Geometry check sheet. Reference: the model listing, model coordinates, mm. A direction names the side the tool comes from. Round coordinates to 2 decimals unless told otherwise and drop trailing zeros. Write each loop counter-clockwise with the first axis right and the second up, starting at its lowest first coordinate (ties: lowest second). Pieces come first, ordered by that corner, then holes.
Item 1: Depth check by flat-ended pin: P1, Ø11.5, axis at x = 80, y = 40, coming from the -Z side; P2, Ø8, axis at x = 72.5, z = 55.5, coming from the -Y side; P3, Ø5, axis at x = 78.5, y = 39.5, coming from the +Z side; P4, Ø13.5, axis at x = 59, y = 77.5, coming from the +Z side. Enter the tip coordinate at first touch or a pass-through.
Item 2: Scan lines: probe 1 along Y at (x, z) = (7, 20.5); probe 2 along Z at (x, y) = (41, 37); probe 3 along Z at (x, y) = (87.5, 22). Record each from-to range of solid material in increasing order.
Item 3: Cross-section at B-B (x = 26). Enter the section's corners in (y, z).
Item 4: Cross-section at A-A (y = 20). Enter the section's corners in (x, z), then the cut area to 4 significant figures.
Item 5: Access from +Z, -Z, +X, -X, +Y, -Y to the whole of each face (thin tool, end or side, straight path). Record for faces 1 (the face through (6.349, 44.957, 15.14)), 2 (the face through (45, 40, 25)), 3 (the face through (60, 20, 13)), 4 (the face through (20, 84, 55)).
Item 6: Draft check along Y on faces 5 (the face through (42.83, 30.24, 15.45)), 6 (the face through (89.619, 18.085, 39.79)), 7 (the face through (80, 0, 13)), 8 (the face through (85, 20, 55)). Enter one of: pulls with the +Y half, pulls with the -Y half, needs draft (parallel to the pull), parting line crosses it, or undercut.
Item 7: Cross-section at D-D (y = 38.5). Enter the section's corners in (x, z), then the cut area to 3 significant figures.
Item 8: Cross-section at C-C (z = 63). Enter the section's corners in (x, y), then the cut area to 3 significant figures.
from build123d import *

# Parameters (mm, degrees)
F1_DEPTH  = 100
F2_R      = 5
F3_DEPTH  = 30
F4_R      = 5
F5_DEPTH  = 20
F6_W      = 60
F6_H      = 40
F7_DEPTH  = 95
F8_W      = 45
F8_H      = 40
F9_DEPTH  = 25
F10_R     = 15
F11_DEPTH = 15
F12_R     = 10
F13_DEPTH = 25


with BuildPart() as f1:
    # F0 (on Right) → F1 (new body)
    with BuildSketch(Plane.YZ):
        Polygon((0, 25), (0, 0), (100, 0), (100, 100), (60, 25), align=None)
    extrude(amount=F1_DEPTH)

    # F2 (on face) → F3 (join)
    with BuildSketch(Plane.XY.offset(25)):
        with Locations((85, 20)):
            Circle(F2_R)
    extrude(amount=F3_DEPTH)

    # F4 (on face) → F5 (cut)
    with BuildSketch(Plane.XY.offset(25)):
        with Locations((7, 40)):
            Circle(F4_R)
        with Locations((80, 40)):
            Circle(F4_R)
    extrude(amount=-F5_DEPTH, mode=Mode.SUBTRACT)

    # F6 (on Front) → F7 (cut)
    with BuildSketch(Plane.XZ):
        with Locations((50, 60)):
            Rectangle(F6_W, F6_H)
    extrude(amount=-F7_DEPTH, mode=Mode.SUBTRACT)

    # F8 (on face) → F9 (cut)
    with BuildSketch(Plane.XY.offset(25)):
        with Locations((37.5, 20)):
            Rectangle(F8_W, F8_H)
    extrude(amount=-F9_DEPTH, mode=Mode.SUBTRACT)

    # F10 (on face) → F11 (cut)
    with BuildSketch(Plane.XY.offset(25)):
        with Locations((45, 40)):
            Circle(F10_R)
    extrude(amount=-F11_DEPTH, mode=Mode.SUBTRACT)

    # F12 (on face) → F13 (join)
    with BuildSketch(Plane.XY.offset(25)):
        with Locations((45, 40)):
            Circle(F12_R)
    extrude(amount=-F13_DEPTH)


solid = f1.part
Resolved:
1. P1: stops at z = 0
1. P2: stops at y = 95
1. P3: stops at z = 5
1. P4: stops at z = 40
2. probe 1: y = 0 to 35, 45 to 100
2. probe 2: z = 0 to 25
2. probe 3: z = 0 to 55
3. outline: (40, 0) - (100, 0) - (100, 100) - (89.33, 80) - (95, 80) - (95, 40) - (68, 40) - (60, 25) - (40, 25) - close
4. outline: (0, 0) - (15, 0) - (15, 25) - (0, 25) - close; (60, 0) - (100, 0) - (100, 25) - (90, 25) - (90, 55) - (80, 55) - (80, 25) - (60, 25) - close
4. area: 1,675 mm2
5. face 1: +Z
5. face 2: +Z, +X, -X, -Y
5. face 3: +Z, -Z, -Y
5. face 4: -Y
6. face 5: undercut
6. face 6: undercut
6. face 7: pulls with the -Y half
6. face 8: needs draft
7. outline: (0, 0) - (15, 0) - (15, 25) - (11.77, 25) - (11.77, 5) - (2.23, 5) - (2.23, 25) - (0, 25) - close; (35.11, 0) - (54.89, 0) - (54.89, 25) - (35.11, 25) - close; (60, 0) - (100, 0) - (100, 25) - (84.77, 25) - (84.77, 5) - (75.23, 5) - (75.23, 25) - (60, 25) - close
7. area: 1,490 mm2
8. outline: (0, 80.27) - (20, 80.27) - (20, 95) - (80, 95) - (80, 80.27) - (100, 80.27) - (100, 100) - (0, 100) - close
8. area: 1,090 mm2
